Here's how the part is built. I have some questions about the finished solid (model axes, mm). A direction names the side the tool comes from. Coordinates: 2 decimals unless noted, no trailing zeros. Write each loop counter-clockwise with the first axis right and the second up, starting at its lowest first coordinate (ties: lowest second). Pieces come first, ordered by that corner, then holes. Notation, with made-up numbers: M -33.75,61.5 L 4.25,61.5 A15 cw 4.25,87.5 Z; hole C 75,-33 d6. An arc over 180 degrees is marked long. Use one line per item in the form item = value. Start each with the question number.
1. On a 3-axis mill with a long thin cutter (end or side, diameter ignored), from which of +Z, -Z, +X, -X, +Y, -Y can I reach the whole of each face in a straight line? I mean faces 4 (the face through (-132.31, 89.85, 6.47)), 5 (the face through (-110, 96, 7.5)), 6 (the face through (-121, 41, 17)), 7 (the face through (-143.01, 57.39, 52.88)). Say none if no direction works.
2. I want a section at A-A, the plane x = -133. List the corners of the cut face in (y, z) for me, plus the area to 3 significant figures.
3. Please list where these lines run through material, in increasing order: line 1 along X through (y, z) = (40.5, 55); line 2 along Z through (x, y) = (-118.5, 88.5); line 3 along Y through (x, z) = (-122, 16). Write a range as [from, to].
4. Thinking about a two-plate mould opening in Y: for faces 1 (the face through (-154.93, 96.97, 6.74)), 2 (the face through (-104.933, 99.098, 3.698)), 3 (the face through (-152.031, 81, 47)), which applies, released by +Y, released by -Y, zero draft, split by the parting line, or undercut?
5. I want a section at B-B, the plane y = 60. List the corners of the cut face in (x, z) for me.
6. I want a section at D-D, the plane x = -156. List the corners of the cut face in (y, z) for me.
7. I'm going to push flat-ended pins straight in: pin 1 Ø12 at (y, z) = (44, 35.5) entering from +X; pin 2 Ø10 at (x, z) = (-124, 56.5) entering from +Y; pin 3 Ø1 at (x, z) = (-142, 24.5) entering from -Y (3 decimals). Where does each tip first touch, or does it pass through?
8. I want a section at C-C, the plane z = 48. List the corners of the cut face in (x, y) for me, plus the area to 3 significant figures.
from build123d import *
from build123d.topology import SkipClean

# Parameters (mm, degrees)
CROQUIS2_R               = 2.5
SALIENTE_EXTRUIR1_DEPTH  = 3
SALIENTE_EXTRUIR2_DEPTH  = 40
CROQUIS4_R               = 2.5
SALIENTE_EXTRUIR3_DEPTH  = 12
CROQUIS7_R               = 12
CORTAR_EXTRUIR1_DEPTH    = 3
CORTAR_EXTRUIR2_DEPTH    = 55.85105
CORTAR_EXTRUIR3_DEPTH    = 40
SALIENTE_EXTRUIR7_DEPTH  = 12
CORTAR_EXTRUIR4_START    = -37.06398
CORTAR_EXTRUIR4_DEPTH    = 34.12796
CROQUIS15_R              = 1
SALIENTE_EXTRUIR8_DEPTH  = 3
SALIENTE_EXTRUIR9_START  = 22
CROQUIS15_2_R            = 1
SALIENTE_EXTRUIR9_DEPTH  = 3
REDONDEO2_R              = 8
CROQUIS32_R              = 2.5
SALIENTE_EXTRUIR14_DEPTH = 6
CROQUIS33_R              = 1.5
SALIENTE_EXTRUIR15_DEPTH = 1.5
SALIENTE_EXTRUIR16_START = -25
SALIENTE_EXTRUIR16_DEPTH = 25


with BuildPart() as part:
    # Croquis2 → Saliente-Extruir1 (new body)
    with BuildSketch(Plane.XY):
        with BuildLine():
            Line((-152.030771759, 47.953613054), (-152.030771759, 99.953613054))
            Line((-152.030771759, 99.953613054), (-112.030771759, 99.953613054))
            Line((-112.030771759, 99.953613054), (-112.030771759, 47.953613054))
            ThreePointArc((-112.030771759, 47.953613054), (-114.449632929, 40.210196563), (-121.030771759, 44.953613054))
            Line((-121.030771759, 44.953613054), (-122.85062293, 49.953613054))
            Line((-122.85062293, 49.953613054), (-141.210920588, 49.953613054))
            Line((-141.210920588, 49.953613054), (-143.030771759, 44.953613054))
            ThreePointArc((-143.030771759, 44.953613054), (-149.611910589, 40.210196563), (-152.030771759, 47.953613054))
        make_face()
        with Locations((-148.030771759, 44.953613054)):
            Circle(CROQUIS2_R, mode=Mode.SUBTRACT)
        with Locations((-116.030771759, 44.953613054)):
            Circle(CROQUIS2_R, mode=Mode.SUBTRACT)
    extrude(amount=SALIENTE_EXTRUIR1_DEPTH)

    # Croquis3 → Saliente-Extruir2 (add)
    with BuildSketch(Plane.ZY.offset(152.030771759)):
        Polygon((3, 99.953613054), (16.75, 99.953613054), (55.851046981, 77.378613054), (42.101046981, 53.56291445), (3, 76.13791445), align=None)
        Polygon((15.379903811, 97.280536842), (4.629903811, 78.660990661), (41.00297077, 57.660990661), (51.75297077, 76.280536842), align=None, mode=Mode.SUBTRACT)
    extrude(amount=-SALIENTE_EXTRUIR2_DEPTH)

    # Croquis4 → Saliente-Extruir3 (add)
    # profile 1 of 2: a face of its own
    with BuildSketch(Plane.XY.offset(3)):
        with BuildLine():
            Line((-152.030771759, 47.953613054), (-152.030771759, 49.953613054))
            Line((-152.030771759, 49.953613054), (-148.030771759, 49.953613054))
            ThreePointArc((-148.030771759, 49.953613054), (-145.794703781, 40.481477099), (-152.030771759, 47.953613054))
        make_face()
        with Locations((-148.030771759, 44.953613054)):
            Circle(CROQUIS4_R, mode=Mode.SUBTRACT)
    # profile 2 of 2: a face of its own
    with BuildSketch(Plane.XY.offset(3)):
        with BuildLine():
            Line((-112.030771759, 49.953613054), (-112.030771759, 47.953613054))
            ThreePointArc((-112.030771759, 47.953613054), (-118.266839736, 40.481477099), (-116.030771759, 49.953613054))
            Line((-116.030771759, 49.953613054), (-112.030771759, 49.953613054))
        make_face()
        with Locations((-116.030771759, 44.953613054)):
            Circle(CROQUIS4_R, mode=Mode.SUBTRACT)
    extrude(amount=SALIENTE_EXTRUIR3_DEPTH)

    # Croquis7 → Cortar-Extruir1 (cut)
    with BuildSketch(Plane(origin=(0, 82.218172547, 47.468684052), x_dir=(1, 0, 0), z_dir=(0, 0.8660254037844387, 0.4999999999999998))):
        with Locations((-149.530771759, 14.320881013)):
            Circle(CROQUIS7_R)
    extrude(amount=-CORTAR_EXTRUIR1_DEPTH, mode=Mode.SUBTRACT)

    # Croquis10 → Cortar-Extruir2 (cut)
    with BuildSketch(Plane(origin=(0, 0, 0), x_dir=(-1, 0, 0), z_dir=(0, 0, -1))):
        with BuildLine():
            Line((152.030771759, 79.953613054), (152.030771759, 49.953613054))
            ThreePointArc((152.030771759, 49.953613054), (145.817568323, 64.953613054), (152.030771759, 79.953613054))
        make_face()
        with BuildLine():
            Line((112.030771759, 79.953613054), (112.030771759, 49.953613054))
            ThreePointArc((112.030771759, 49.953613054), (118.243975195, 64.953613054), (112.030771759, 79.953613054))
        make_face()
    extrude(amount=-CORTAR_EXTRUIR2_DEPTH, mode=Mode.SUBTRACT)

    # Croquis11 → Cortar-Extruir3 (cut)
    with BuildSketch(Plane.ZY.offset(152.030771759)):
        Polygon((12.839840301, 97.881017789), (2.839840301, 80.560509714), (1.540802195, 81.310509714), (11.540802195, 98.631017789), align=None)
    extrude(amount=-CORTAR_EXTRUIR3_DEPTH, mode=Mode.SUBTRACT)

    # Croquis12 → Saliente-Extruir7 (add)
    with SkipClean():  # the faces are left unmerged after this step: merging them gives an invalid solid
        with BuildSketch(Plane.XY.offset(3)):
            with BuildLine():
                Line((-152.030771759, 49.953613054), (-148.030771759, 49.953613054))
                ThreePointArc((-148.030771759, 49.953613054), (-144.495237853, 48.48914696), (-143.030771759, 44.953613054))
                Line((-143.030771759, 44.953613054), (-141.530771759, 49.074829183))
                Line((-141.530771759, 49.074829183), (-141.530771759, 76.13791445))
                Line((-141.530771759, 76.13791445), (-149.005472808, 76.13791445))
                ThreePointArc((-149.005472808, 76.13791445), (-145.957755776, 62.518865142), (-152.030771759, 49.953613054))
            make_face()
            with BuildLine():
                Line((-121.030771759, 44.953613054), (-122.530771759, 49.074829183))
                Line((-122.530771759, 49.074829183), (-122.530771759, 76.13791445))
                Line((-122.530771759, 76.13791445), (-115.05607071, 76.13791445))
                ThreePointArc((-115.05607071, 76.13791445), (-118.103787742, 62.518865142), (-112.030771759, 49.953613054))
                Line((-112.030771759, 49.953613054), (-116.030771759, 49.953613054))
                ThreePointArc((-116.030771759, 49.953613054), (-119.566305665, 48.48914696), (-121.030771759, 44.953613054))
            make_face()
        extrude(amount=SALIENTE_EXTRUIR7_DEPTH)

    # Croquis14 → Cortar-Extruir4 (cut)
    with BuildSketch(Plane.ZY.offset(152.030771759).offset(CORTAR_EXTRUIR4_START)):
        Polygon((15.379903811, 97.280536842), (51.88287458, 76.205536842), (41.13287458, 57.585990661), (4.629903811, 78.660990661), align=None)
    extrude(amount=CORTAR_EXTRUIR4_DEPTH, mode=Mode.SUBTRACT)

    # Croquis15 → Saliente-Extruir8 (add)
    with BuildSketch(Plane(origin=(-141.530771759, 0, 0), x_dir=(0, 0, -1), z_dir=(1, 0, 0))):
        with BuildLine():
            Line((-15, 69.209711219), (-15, 49.709711219))
            Line((-15, 49.709711219), (-17, 49.709711219))
            Line((-17, 49.709711219), (-17, 31.865013093))
            Line((-17, 31.865013093), (-50.633644315, 31.865013093))
            Line((-50.633644315, 31.865013093), (-62.036793098, 31.865013093))
            ThreePointArc((-62.036793098, 31.865013093), (-64.120396014, 42.938683324), (-58.500710752, 52.705295379))
            Line((-58.500710752, 52.705295379), (-47.019992598, 62.269965257))
            Line((-47.019992598, 62.269965257), (-42.019992598, 53.609711219))
            Line((-42.019992598, 53.609711219), (-15, 69.209711219))
        make_face()
        with Locations((-48.09937995, 40.220311696)):
            Circle(CROQUIS15_R, mode=Mode.SUBTRACT)
    extrude(amount=-SALIENTE_EXTRUIR8_DEPTH)

    # Croquis15<2> → Saliente-Extruir9 (add)
    with BuildSketch(Plane(origin=(-141.530771759, 0, 0), x_dir=(0, 0, -1), z_dir=(1, 0, 0)).offset(SALIENTE_EXTRUIR9_START)):
        with BuildLine():
            Line((-15, 69.209711219), (-15, 49.709711219))
            Line((-15, 49.709711219), (-17, 49.709711219))
            Line((-17, 49.709711219), (-17, 31.865013093))
            Line((-17, 31.865013093), (-50.633644315, 31.865013093))
            Line((-50.633644315, 31.865013093), (-62.036793098, 31.865013093))
            ThreePointArc((-62.036793098, 31.865013093), (-64.120396014, 42.938683324), (-58.500710752, 52.705295379))
            Line((-58.500710752, 52.705295379), (-47.019992598, 62.269965257))
            Line((-47.019992598, 62.269965257), (-42.019992598, 53.609711219))
            Line((-42.019992598, 53.609711219), (-15, 69.209711219))
        make_face()
        with Locations((-48.09937995, 40.220311696)):
            Circle(CROQUIS15_2_R, mode=Mode.SUBTRACT)
    extrude(amount=-SALIENTE_EXTRUIR9_DEPTH)

    # Redondeo2
    redondeo2_edges = [part.edges().sort_by_distance(p)[0] for p in [
        (-132.030771759, 99.953613054, 16.75),
    ]]
    fillet(redondeo2_edges, radius=REDONDEO2_R)

    # Croquis32 → Saliente-Extruir14 (add)
    with BuildSketch(Plane(origin=(0, 0, 0), x_dir=(-1, 0, 0), z_dir=(0, 0, -1))):
        with BuildLine():
            Line((112.030771759, 99.953613054), (107.030771759, 99.953613054))
            ThreePointArc((107.030771759, 99.953613054), (104.909451415, 99.074933397), (104.030771759, 96.953613054))
            Line((104.030771759, 96.953613054), (104.030771759, 94.953613054))
            ThreePointArc((104.030771759, 94.953613054), (104.909451415, 92.83229271), (107.030771759, 91.953613054))
            Line((107.030771759, 91.953613054), (112.030771759, 91.953613054))
            Line((112.030771759, 91.953613054), (112.030771759, 99.953613054))
        make_face()
        with Locations((108.030771759, 95.953613054)):
            Circle(CROQUIS32_R, mode=Mode.SUBTRACT)
    saliente_extruir14 = extrude(amount=-SALIENTE_EXTRUIR14_DEPTH)

    # Croquis33 → Saliente-Extruir15 (add)
    with BuildSketch(Plane.XY.offset(6)):
        with BuildLine():
            Line((-112.030771759, 99.953613054), (-107.030771759, 99.953613054))
            ThreePointArc((-107.030771759, 99.953613054), (-104.909451415, 99.074933397), (-104.030771759, 96.953613054))
            Line((-104.030771759, 96.953613054), (-104.030771759, 94.953613054))
            ThreePointArc((-104.030771759, 94.953613054), (-104.909451415, 92.83229271), (-107.030771759, 91.953613054))
            Line((-107.030771759, 91.953613054), (-112.030771759, 91.953613054))
            Line((-112.030771759, 91.953613054), (-112.030771759, 99.953613054))
        make_face()
        with Locations((-108.030771759, 95.953613054)):
            Circle(CROQUIS33_R, mode=Mode.SUBTRACT)
    saliente_extruir15 = extrude(amount=SALIENTE_EXTRUIR15_DEPTH)

    # Simetría1: Saliente-Extruir14, Saliente-Extruir15 across plane
    add(saliente_extruir14.mirror(Plane(origin=(-132.030771759, 0, 0), x_dir=(0, 0, 1), z_dir=(1, 0, 0))))
    add(saliente_extruir15.mirror(Plane(origin=(-132.030771759, 0, 0), x_dir=(0, 0, 1), z_dir=(1, 0, 0))))

    # Croquis36 → Saliente-Extruir16 (add)
    with BuildSketch(Plane.ZY.offset(144.530771759).offset(SALIENTE_EXTRUIR16_START)):
        with BuildLine():
            Line((57.036793098, 31.865013093), (62.036793098, 31.865013093))
            ThreePointArc((62.036793098, 31.865013093), (61.45100666, 30.450799531), (60.036793098, 29.865013093))
            Line((60.036793098, 29.865013093), (59.036793098, 29.865013093))
            Line((59.036793098, 29.865013093), (57.036793098, 31.865013093))
        make_face()
    extrude(amount=SALIENTE_EXTRUIR16_DEPTH)


solid = part.part
Answer list:
q1.face_4 = +X, -X
q1.face_5 = +Z, +X, +Y
q1.face_6 = +X, -X, -Y
q1.face_7 = +Z, +X, -X
q2.outline = M 29.87,59.04 L 31.87,57.04 L 31.87,62.04 A2 ccw 29.87,60.04 Z; M 49.95,0 L 99.95,0 L 99.95,14.61 A8 ccw 98.88,18.61 L 77.38,55.85 L 53.56,42.1 L 76.14,3 L 49.95,3 Z; hole M 57.59,41.13 L 78.66,4.63 L 97.28,15.38 L 76.21,51.88 Z; hole M 80.56,2.84 L 81.31,1.54 L 98.63,11.54 L 97.88,12.84 Z
q2.area = 626 mm²
q3.line_1 = [-144.53, -141.53], [-122.53, -119.53]
q3.line_2 = [0, 5.69], [7.42, 10.31], [30.59, 36.59]
q3.line_3 = [49.71, 72.1], [96.92, 99.83]
q4.face_1 = undercut
q4.face_2 = released by +Y
q4.face_3 = zero draft
q5.outline = M -146.4,0 L -117.66,0 L -117.66,15 L -119.53,15 L -119.53,30.95 L -117.66,30.95 L -117.66,36.95 L -146.4,36.95 L -146.4,30.95 L -144.53,30.95 L -144.53,15 L -146.4,15 Z; M -146.4,42.53 L -117.66,42.53 L -117.66,45.82 L -119.53,45.82 L -119.53,49.74 L -122.53,49.74 L -122.53,45.82 L -141.53,45.82 L -141.53,49.74 L -144.53,49.74 L -144.53,45.82 L -146.4,45.82 Z; hole M -141.53,3 L -122.53,3 L -122.53,30.95 L -141.53,30.95 Z
q6.outline = M 91.95,0 L 93.45,0 L 93.45,6 L 94.45,6 L 94.45,7.5 L 91.95,7.5 Z; M 97.45,6 L 98.45,6 L 98.45,0 L 99.95,0 L 99.95,7.5 L 97.45,7.5 Z
q7.pin_1 = -119.53
q7.pin_2 = 79.89
q7.pin_3 = 31.865
q8.outline = M -152.03,79.95 A21.21 cw -150.66,78.45 L -113.4,78.45 A21.21 cw -112.03,79.95 L -112.03,81.91 L -152.03,81.91 Z; M -146.31,69.48 A21.21 cw -145.85,63.78 L -118.21,63.78 A21.21 cw -117.76,69.48 Z; M -144.53,31.87 L -141.53,31.87 L -141.53,39.23 L -144.53,39.23 Z; M -144.53,41.22 L -141.53,41.22 L -141.53,61.45 L -144.53,61.45 Z; M -122.53,31.87 L -119.53,31.87 L -119.53,39.23 L -122.53,39.23 Z; M -122.53,41.22 L -119.53,41.22 L -119.53,61.45 L -122.53,61.45 Z
q8.area = 461 mm²
